Model file for the job. Use its own axes, mm. A direction names the side the tool comes from. Coordinates: 2 decimals unless noted, no trailing zeros. Write each loop counter-clockwise with the first axis right and the second up, starting at its lowest first coordinate (ties: lowest second). Pieces come first, ordered by that corner, then holes. Notation, with made-up numbers: M -34,73.5 L -3,73.5 A26 cw -3,87.5 Z; hole C 80.5,-28.75 d8. An arc over 180 degrees is marked long. Put each result on its own line as item: value. Start each with the question number.
Q1. Drill centre lines: line 1 along Y through (x, z) = (-91, -1.5); line 2 along X through (y, z) = (-79.5, 72.5); line 3 along X through (y, z) = (-46.5, 25). Where is each one in solid material? Low to high.
Q2. Cut at A-A (z = 26.5). Write the cut outline in (x, y).
Q3. Pull direction X, two halves, no side cores. Call faces 4 (the flat face through (-110, -110, 88.9)), 5 (the flat face through (12.7, -174, 38)), 6 (the conical face through (-167.89, -6.44, 38.35)): pulls with the +X half, pulls with the -X half, needs draft (parallel to the pull), parting line crosses it, or undercut.
Q4. Which spindle directions (+Z, -Z, +X, -X, +Y, -Y) get a long thin tool onto all of the face, cutting with end or side? Do faces 1 (the flat face through (-104, -104, 76.2)), 2 (the conical face through (-127.539, -124.765, -0.004)), 3 (the flat face through (-174, -12.7, 38)). Say none if no direction does.
Q5. Drop flat-ended pins along their axis: pin 1 (1.5 mm diameter, centred on x = -153.5, y = -80.5, fed in from +Z); pin 2 (5 mm diameter, centred on y = -165, z = 18.5, fed in from +X); pin 3 (3 mm diameter, centred on x = -83, z = 37.5, fed in from -Y); pin 4 (12 mm diameter, centred on x = -123, y = -122.5, fed in from +Z). Give the stop position or say it passes through.
```python
from build123d import *

# Parameters (mm, degrees)
F1_ANGLE = 90
F2_R     = 6.35
F3_DEPTH = 12.7
F3_TAPER = 5
F4_R     = 6.35
F5_DEPTH = 12.7
F5_TAPER = 5


# Not quite as in the source:
# - a feature names something its author has since deleted; it is built from what else it names


with BuildPart() as f1:
    # F0 (on Front) → F1 (revolve)
    with BuildSketch(Plane.XZ):
        with BuildLine():
            Line((-190.5, 0), (-177.7999999529, -0.0040913673))
            ThreePointArc((-177.7999999529, -0.0040913673), (-177.6863527462, -6.3561031883), (-177.3458485559, -12.7))
            Line((-177.3458485559, -12.7), (-164.6108137396, -12.7))
            ThreePointArc((-164.6108137396, -12.7), (-164.9776583118, -6.354703608), (-165.1, 1.06856e-05))
            ThreePointArc((-165.1, 1.06856e-05), (-160.3732216696, 39.2229495488), (-146.4635449523, 76.2))
            Line((-146.4635449523, 76.2), (-160.6437051366, 76.2))
            ThreePointArc((-160.6437051366, 76.2), (-157.4396201151, 82.6172259157), (-153.9793167929, 88.9))
            Line((-153.9793167929, 88.9), (-168.4845393501, 88.9))
            ThreePointArc((-168.4845393501, 88.9), (-184.9142432943, 45.792713688), (-190.5, 0))
        make_face()
    revolve(axis=Axis((0, 0, 38.1), (0, 0, 1)), revolution_arc=F1_ANGLE)

    # F2 (on face) → F3 (join)
    with BuildSketch(Plane.YZ):
        with Locations((-173.669888006, 38.1)):
            Circle(F2_R)
    extrude(amount=F3_DEPTH, taper=F3_TAPER)

    # F4 (on face) → F5 (cut)
    with BuildSketch(Plane(origin=(0, 0, 0), x_dir=(-1, 0, 0), z_dir=(0, 1, 0))):
        with Locations((173.669888006, 38.1)):
            Circle(F4_R)
    extrude(amount=-F5_DEPTH, taper=F5_TAPER, mode=Mode.SUBTRACT)


solid = f1.part
```
Computed values:
1. line 1: -152.74 to -137.75
1. line 2: -157.21 to -125.23
1. line 3: -183.04 to -156.43
2. outline: M -188.65,0 A188.65 ccw 0,-188.65 L 0,-162.96 A162.96 cw -162.96,0 Z
3. face 4: needs draft
3. face 5: pulls with the +X half
3. face 6: undercut
4. face 1: +X, +Y
4. face 2: -Z, -X, -Y
4. face 3: +Y
5. pin 1: z = 80.67
5. pin 2: x = 0
5. pin 3: y = -168.12
5. pin 4: z = 88.9
